```python
from build123d import *

# Parameters (mm, degrees)
SKETCH1_W           = 20
SKETCH1_H           = 20
BOSS_EXTRUDE1_DEPTH = 5
SKETCH2_R           = 5
CUT_EXTRUDE1_DEPTH  = 2
SKETCH3_R           = 1
CUT_EXTRUDE2_DEPTH  = 2
FILLET1_R           = 1


with BuildPart() as part:
    # Sketch1 → Boss-Extrude1 (new body)
    with BuildSketch(Plane(origin=(0, 0, 0), x_dir=(1, 0, 0), z_dir=(0, 1, 0))):
        Rectangle(SKETCH1_W, SKETCH1_H)
    extrude(amount=BOSS_EXTRUDE1_DEPTH)

    # Sketch2 → Cut-Extrude1 (cut)
    with BuildSketch(Plane(origin=(0, 5, 0), x_dir=(1, 0, 0), z_dir=(0, 1, 0))):
        Circle(SKETCH2_R)
    extrude(amount=-CUT_EXTRUDE1_DEPTH, mode=Mode.SUBTRACT)

    # Sketch3 → Cut-Extrude2 (cut)
    with BuildSketch(Plane.XZ):
        Circle(SKETCH3_R)
    extrude(amount=-CUT_EXTRUDE2_DEPTH, mode=Mode.SUBTRACT)

    # Fillet1
    fillet1_edges = [part.edges().sort_by_distance(p)[0] for p in [
        (-1, 2, 0),
    ]]
    fillet(fillet1_edges, radius=FILLET1_R)


solid = part.part
```
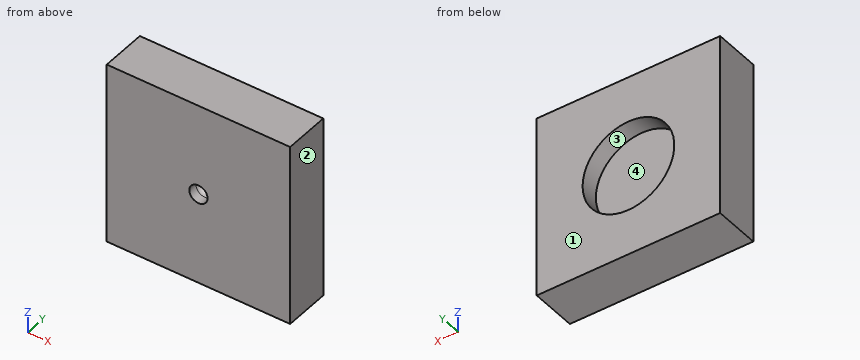
CAD build for the part. Positions are in the model's coordinates, mm. Face numbers are marked on the shaded views. Coordinates: 2 decimals unless noted, no trailing zeros. Write each loop counter-clockwise with the first axis right and the second up, starting at its lowest first coordinate (ties: lowest second). Pieces come first, ordered by that corner, then holes. Notation, with made-up numbers: (24.25, 55.25) -> (82.25, 55.25) arc R28 cw to (82.25, 90.25) -> close; hole circle Ø1 at (86.5, 69). An arc over 180 degrees is marked (long way). Use CSV: the item, a comma, the result in double quotes. Start each with the question number.
Item 1: Band-saw the part on B-B, the plane y = 4.6. Write the cut outline in (x, z).
Item 2: Two-plate mould, pull along X, no slides. Class the marked faces 1, 2, 3 and 4: +X half, -X half, draft (parallel to the pull), parting line (faces both ways), or undercut.
Item 3: Wall check: probe 1 along Z at (x, y) = (0, 0.4); probe 2 along Z at (x, y) = (0, 3.95). Give the ranges that are in metal, low to high.
Item 4: Band-saw the part on D-D, the plane z = 2.5. Write the cut outline in (x, y).
Item 5: Drop flat-ended pins along their axis: P1, Ø3, axis at x = 0, z = 0, coming from the +Y side; P2, Ø11, axis at x = -2, z = 1, coming from the +Y side. Give the stop position or say it passes through.
Item 6: Band-saw the part on C-C, the plane z = 0. Write the cut outline in (x, y), plus the area to 3 significant figures.
Item 7: Band-saw the part on A-A, the plane x = 0. Write the cut outline in (y, z), plus the area to 3 significant figures.
Response values:
1,outline,"(-10, -10) -> (10, -10) -> (10, 10) -> (-10, 10) -> close; hole circle Ø10 at (0, 0)"
2,face 1,"draft"
2,face 2,"+X half"
2,face 3,"undercut"
2,face 4,"undercut"
3,probe 1,"z = -10 to -1, 1 to 10"
3,probe 2,"z = -10 to -5, 5 to 10"
4,outline,"(-10, 0) -> (10, 0) -> (10, 5) -> (4.33, 5) -> (4.33, 3) -> (-4.33, 3) -> (-4.33, 5) -> (-10, 5) -> close"
5,P1,"stops at y = 3"
5,P2,"stops at y = 5"
6,outline,"(-10, 0) -> (-1, 0) -> (-1, 1) arc R1 cw to (1, 1) -> (1, 0) -> (10, 0) -> (10, 5) -> (5, 5) -> (5, 3) -> (-5, 3) -> (-5, 5) -> (-10, 5) -> close"
6,area,"76.4 mm2"
7,outline,"(0, -10) -> (5, -10) -> (5, -5) -> (3, -5) -> (3, 5) -> (5, 5) -> (5, 10) -> (0, 10) -> (0, 1) -> (1, 1) arc R1 cw to (1, -1) -> (0, -1) -> close"
7,area,"76.4 mm2"
